Autodesk Inventor part; units mm, degrees
ref_plane "YZ Plane" through (0, 0, 0) normal (1, 0, 0) x (0, 1, 0)
ref_plane "XZ Plane" through (0, 0, 0) normal (0, 1, 0) x (-1, 0, 0)
ref_plane "XY Plane" through (0, 0, 0) normal (0, 0, 1) x (1, 0, 0)
sketch "スケッチ1" plane through (0, 0, 0) normal (0, 0, 1) x (1, 0, 0)
  line L0 (34.5, -2.7) -> (15.5, -2.7)
  line L1 (50, -5) -> (0, -5)
  line L2 (12, -5) -> (12, 5)
  circle A0 centre (44, 0) radius 2.75
  circle A1 centre (6, 0) radius 2.75
  line L3 (50, -5) -> (50, 5)
  line L4 (0, 5) -> (50, 5)
  line L5 (0, -5) -> (0, 5)
  line L6 (50, -5) -> (0, -5)
  line L7 (0, -5) -> (160, -5)
  line L8 (160, -5) -> (160, 45)
  line L9 (160, 45) -> (0, 45)
  line L10 (0, 45) -> (0, -5)
  point P0 (0, 0)
  dimension "d0" = 160
  dimension "d1" = 50
extrude "押し出し1" add sketch "スケッチ1" along normal blind 10
The listing builds one solid part. Answer for the finished solid, in the listing's coordinates (mm). Round coordinates to 2 decimals unless told otherwise and drop trailing zeros. Write each loop counter-clockwise with the first axis right and the second up, starting at its lowest first coordinate (ties: lowest second). Pieces come first, ordered by that corner, then holes. Notation, with made-up numbers: (12, 65) - (46, 65) arc R15 cw to (46, 83) - close; hole circle Ø7 at (31.25, 70.25). An arc over 180 degrees is marked (long way). Use one line per item in the form item = value. Start each with the question number.
Item 1: A cutting plane is placed at A-A (y = 0). Write down the section's boundary in (x, z), plus the area to 3 significant figures.
Item 2: Determine the mould class of faces 1 (the flat face through (160, 20, 5)), 2 (the flat face through (81, -5, 5)), 3 (the cylindrical face through (8.54, 1.05, 4.93)) for opening direction X: +X half, -X half, draft (parallel to the pull), parting line (faces both ways), or undercut.
Item 3: A cutting plane is placed at B-B (x = 44). Write down the section's boundary in (y, z), plus the area to 3 significant figures.
Item 4: Find the intervals of material crossed by line 1 (Y direction, x = 6, z = 8); line 2 (X direction, y = -2, z = 3.5), in increasing order. Write a range as [from, to].
The answers:
q1.outline = (0, 0) - (3.25, 0) - (3.25, 10) - (0, 10) - close; (8.75, 0) - (41.25, 0) - (41.25, 10) - (8.75, 10) - close; (46.75, 0) - (160, 0) - (160, 10) - (46.75, 10) - close
q1.area = 1,490 mm^2
q2.face_1 = +X half
q2.face_2 = draft
q2.face_3 = undercut
q3.outline = (-5, 0) - (-2.75, 0) - (-2.75, 10) - (-5, 10) - close; (2.75, 0) - (45, 0) - (45, 10) - (2.75, 10) - close
q3.area = 445 mm^2
q4.line_1 = [-5, -2.75], [2.75, 45]
q4.line_2 = [0, 4.11], [7.89, 42.11], [45.89, 160]
